from build123d import *

# Parameters (mm, degrees)
SKETCH1_R       = 10
BODY_DEPTH      = 25
SKETCH2_R       = 4
BORE_LOW_DEPTH  = 12
SKETCH3_R       = 2
BORE_HIGH_DEPTH = 10


with BuildPart() as part:
    # Sketch1 → Body (new body)
    with BuildSketch(Plane.XY):
        Circle(SKETCH1_R)
    extrude(amount=BODY_DEPTH)

    # Sketch2 → Bore_low (cut)
    with BuildSketch(Plane.XY):
        Circle(SKETCH2_R)
    extrude(amount=BORE_LOW_DEPTH, mode=Mode.SUBTRACT)

    # Sketch3 → Bore_high (cut)
    with BuildSketch(Plane.XY.offset(15)):
        Circle(SKETCH3_R)
    extrude(amount=BORE_HIGH_DEPTH, mode=Mode.SUBTRACT)


solid = part.part
Verification items for the finished model (mm, model axes). A direction names the side the tool comes from. Round coordinates to 2 decimals unless told otherwise and drop trailing zeros. Order: outer loops, then holes, each group sorted by start corner. A loop starts at its lowest first (then second) coordinate and runs counter-clockwise, first axis right, second up.
1. Section check D-D on z = 13.25. Record the cut outline in (x, y), then the cut area to 3 significant figures.
Final values:
outline: circle Ø20 at (0, 0)
area: 314 mm2
2. Go/stop test with flat-tipped pins: P1, Ø3, axis at x = 6.5, z = 13, coming from the -Y side; P2, Ø2.5, axis at x = 0, y = 0, coming from the -Z side; P3, Ø4, axis at x = -2.5, z = 10.5, coming from the +Y side. Record where each tip stops, or that it passes through.
Final values:
P1: stops at y = -8.66
P2: stops at z = 12
P3: stops at y = 9.99
3. Release check for a two-part mould opening along X. For faces 4 (the cylindrical face through (0, -2, 20)), 5 (the cylindrical face through (-2.17, -9.76, 12.32)), 6 (the flat face through (-0.1, 2.4, 25)) record: +X half, -X half, draft (parallel to the pull), parting line (faces both ways), or undercut.
Final values:
face 4: undercut
face 5: parting line
face 6: draft
4. Thickness scan on L1, parallel to Y at x = 0, z = 7.75; L2, parallel to X at y = -0.25, z = 11.5; L3, parallel to Y at x = -0.5, z = 22.25. Record the ranges inside material, lowest first.
Final values:
L1: y = -10 to -4, 4 to 10
L2: x = -10 to -3.99, 3.99 to 10
L3: y = -9.99 to -1.94, 1.94 to 9.99
5. Access from +Z, -Z, +X, -X, +Y, -Y to the whole of each face (thin tool, end or side, straight path). Record for faces 1 (the cylindrical face through (-0.867, -3.905, 5.916)), 2 (the flat face through (-0.1, -4.3, 0)), 3 (the flat face through (0, 0, 15)).
Final values:
face 1: -Z
face 2: -Z, +X, -X, +Y, -Y
face 3: +Z
6. Section check A-A on y = 0. Record the cut outline in (x, z).
Final values:
outline: (-10, 0) - (-4, 0) - (-4, 12) - (4, 12) - (4, 0) - (10, 0) - (10, 25) - (2, 25) - (2, 15) - (-2, 15) - (-2, 25) - (-10, 25) - close
7. Section check C-C on z = 10. Record the cut outline in (x, y).
Final values:
outline: circle Ø20 at (0, 0); hole circle Ø8 at (0, 0)
